Geometry check sheet. Reference: drawing and pictorial views, mm from the part's lowest x, y, z. Give positions to 0.01 mm unless a question says otherwise; leave off trailing zeros. Order: outer loops, then holes, each group sorted by start corner. A loop starts at its lowest first (then second) coordinate and runs counter-clockwise, first axis right, second up. Notation, with made-up numbers: (26, 53.25) - (34, 53.25) arc R26 ccw to (34, 71.25) - close; hole circle Ø6 at (-28, 71). An arc over 180 degrees is marked (long way). Answer as a JSON object with one key per item and string values.
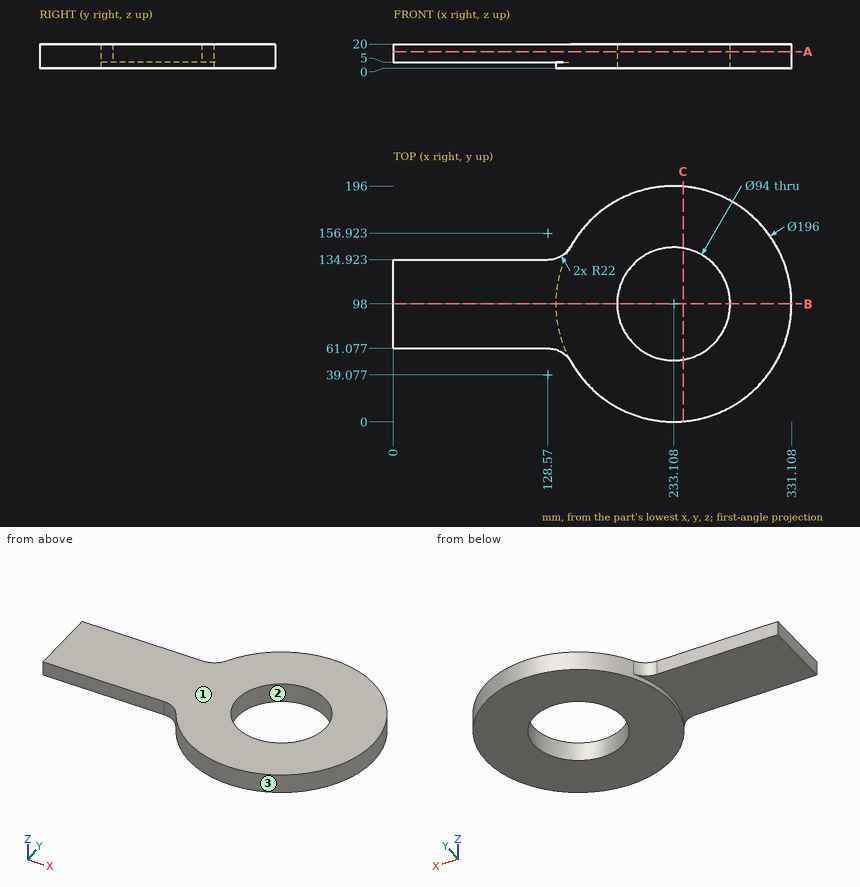
(1) Release check for a two-part mould opening along X. For the marked faces 1, 2 and 3 record: pulls with the +X half, pulls with the -X half, needs draft (parallel to the pull), parting line crosses it, or undercut.
Computed values:
{"face 1": "needs draft", "face 2": "undercut", "face 3": "parting line crosses it"}
(2) Material ranges on line 1 along Z through (x, y) = (109, 134.5); line 2 along Y through (x, z) = (19, 12.5); line 3 along X through (y, z) = (105.5, 11.25) (1 decimal), recorded low to high. Write a range as [from, to].
Computed values:
{"line 1": "z = [5, 20]", "line 2": "y = [61.08, 134.92]", "line 3": "x = [0, 186.7], [279.5, 330.8]"}
(3) Section check C-C (x = 241). Record the cut outline in (y, z), then the cut area to 3 significant figures.
Computed values:
{"outline": "(0.32, 0) - (51.67, 0) - (51.67, 20) - (0.32, 20) - close; (144.33, 0) - (195.68, 0) - (195.68, 20) - (144.33, 20) - close", "area": "2,050 mm²"}
(4) Section check B-B (y = 98). Record the cut outline in (x, z), then the cut area to 3 significant figures.
Computed values:
{"outline": "(0, 5) - (135.11, 5) - (135.11, 0) - (186.11, 0) - (186.11, 20) - (0, 20) - close; (280.11, 0) - (331.11, 0) - (331.11, 20) - (280.11, 20) - close", "area": "4,070 mm²"}
(5) Section check A-A (z = 13.75). Record the cut outline in (x, y) (1 decimal).
Computed values:
{"outline": "(0, 61.1) - (128.6, 61.1) arc R22 cw to (147.7, 49.9) arc R98 ccw (long way) to (147.7, 146.1) arc R22 cw to (128.6, 134.9) - (0, 134.9) - close; hole circle Ø94 at (233.1, 98)"}
(6) Gauge pin test, flat ends, axial feed: pin 1 Ø8 at (y, z) = (29.5, 16.5) entering from +X; pin 2 Ø12 at (x, z) = (82, 11) entering from +Y; pin 3 Ø8 at (y, z) = (148, 4) entering from -X (1 decimal). Record the tip position at first contact, or that the pin passes through.
Computed values:
{"pin 1": "stops at x = 306.89", "pin 2": "stops at y = 134.92", "pin 3": "stops at x = 146.5"}
